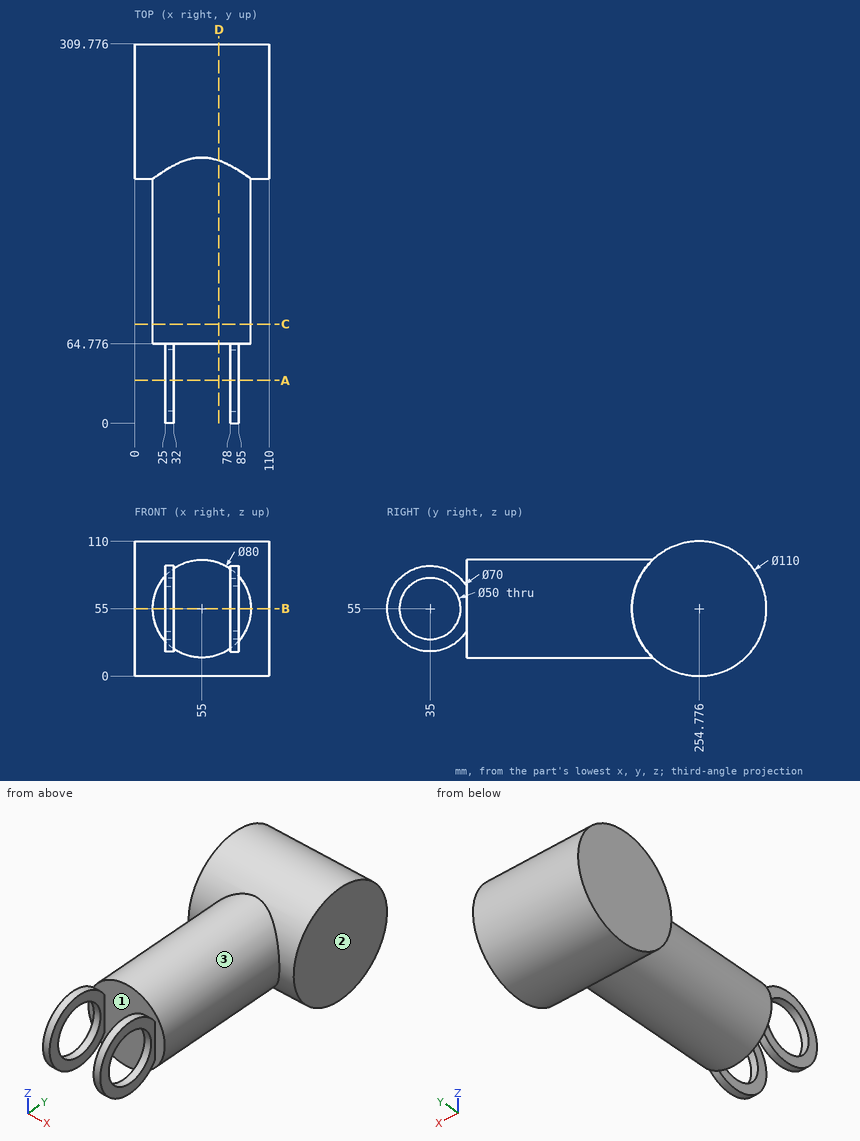
Verification items for this drawing (mm, ordinates from the low corner). Coordinates: 2 decimals unless noted, no trailing zeros. Order: outer loops, then holes, each group sorted by start corner. A loop starts at its lowest first (then second) coordinate and runs counter-clockwise, first axis right, second up. Notation, with made-up numbers: (-15, 88.5) - (40, 88.5) arc R16 cw to (40, 104.5) - close; hole circle Ø2 at (-24, 54.25). An arc over 180 degrees is marked (long way). Answer in a Markdown table with one row per item. Add a question column.
1. Section check A-A (y = 35). Enter the section's corners in (x, z).
2. Section check D-D (x = 69). Enter the section's corners in (y, z).
3. Section check C-C (y = 81). Enter the section's corners in (x, z), plus the area to 3 significant figures.
4. Gauge pin test, flat ends, axial feed: pin 1 Ø3 at (x, z) = (46.5, 53.5) entering from -Y; pin 2 Ø3 at (x, y) = (31, 188.5) entering from -Z; pin 3 Ø5 at (x, y) = (37.5, 152) entering from -Z. Record the tip position at first contact, or that the pin passes through.
5. Draft check along X on the marked faces 1, 2 and 3. Enter one of: +X half, -X half, draft (parallel to the pull), parting line (faces both ways), or undercut.
6. Material ranges on L1, parallel to Y at x = 82, z = 55; L2, parallel to X at y = 45.5, z = 25; L3, parallel to Y at x = 5, z = 45, recorded low to high. Write a range as [from, to].
7. Section check B-B (z = 55). Enter the section's corners in (x, y).
Data:
| question | item | result |
|---|---|---|
| 1 | outline | (25, 20) - (32, 20) - (32, 30) - (25, 30) - close; (25, 80) - (32, 80) - (32, 90) - (25, 90) - close; (78, 20) - (85, 20) - (85, 30) - (78, 30) - close; (78, 80) - (85, 80) - (85, 90) - (78, 90) - close |
| 2 | outline | (64.78, 17.53) - (214.51, 17.53) arc R55 ccw (long way) to (214.51, 92.47) - (64.78, 92.47) - close |
| 3 | outline | circle Ø80 at (55, 55) |
| 3 | area | 5,030 mm² |
| 4 | pin 1 | stops at y = 64.78 |
| 4 | pin 2 | stops at z = 21.93 |
| 4 | pin 3 | stops at z = 17.92 |
| 5 | face 1 | undercut |
| 5 | face 2 | +X half |
| 5 | face 3 | parting line |
| 6 | L1 | y = [0, 10], [60, 309.78] |
| 6 | L2 | x = [25, 32], [78, 85] |
| 6 | L3 | y = [200.69, 308.86] |
| 7 | outline | (0, 199.78) - (15, 199.78) - (15, 64.78) - (25, 64.78) - (25, 60) - (32, 60) - (32, 64.78) - (78, 64.78) - (78, 60) - (85, 60) - (85, 64.78) - (95, 64.78) - (95, 199.78) - (110, 199.78) - (110, 309.78) - (0, 309.78) - close; (25, 0) - (32, 0) - (32, 10) - (25, 10) - close; (78, 0) - (85, 0) - (85, 10) - (78, 10) - close |
